Input: part model. Units: mm. Frame: model coordinates. Round coordinates to 2 decimals unless told otherwise and drop trailing zeros. Order: outer loops, then holes, each group sorted by start corner. A loop starts at its lowest first (then second) coordinate and runs counter-clockwise, first axis right, second up. Notation, with made-up numbers: (34, -29.75) -> (71, -29.75) arc R13 cw to (71, -11.75) -> close; hole circle Ø3 at (77.25, 69.25). An arc over 180 degrees is marked (long way). Use a Markdown table: item, result.
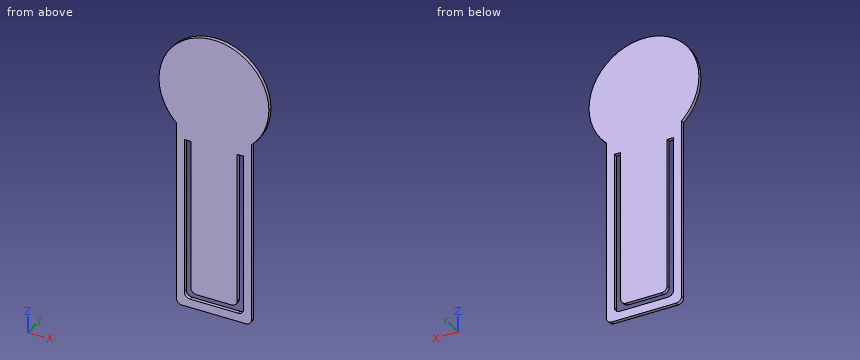
from build123d import *

# Parameters (mm, degrees)
F1_DEPTH = 1
F2_R     = 1.5
F3_R     = 1.5
F4_R     = 1.5
F5_R     = 1.5


with BuildPart() as f1:
    # F0 (on Front) → F1 (new body)
    with BuildSketch(Plane.XZ):
        with BuildLine():
            ThreePointArc((-12.582927, 26.823092), (-9.070294, 31.806561), (-7.831176, 37.776329))
            ThreePointArc((-7.831176, 37.776329), (-28.798743, 51.538165), (-33.082927, 26.826371))
            Line((-33.082927, 26.826371), (-12.582927, 26.826371))
            Line((-12.582927, 26.826371), (-12.582927, 26.823092))
        make_face()
        with BuildLine():
            Line((-12.582927, 26.826371), (-33.082927, 26.826371))
            ThreePointArc((-33.082927, 26.826371), (-22.833574, 22.776329), (-12.582927, 26.823092))
            Line((-12.582927, 26.823092), (-12.582927, 26.826371))
        make_face()
        with BuildLine():
            ThreePointArc((-12.582927, 26.823092), (-22.833574, 22.776329), (-33.082927, 26.826371))
            Line((-33.082927, 26.826371), (-33.082927, -23.173629))
            Line((-33.082927, -23.173629), (-12.582927, -23.173629))
            Line((-12.582927, -23.173629), (-12.582927, 26.823092))
        make_face()
        Polygon((-30.924927, -19.130884), (-30.924927, 22.876894), (-29.146819, 22.876894), (-29.146819, -19.130884), (-16.490985, -19.130884), (-16.490985, 23.022754), (-14.740985, 23.022754), (-14.740985, -19.130884), (-14.740985, -20.88121), (-16.490985, -20.88121), (-29.146819, -20.88121), (-30.924927, -20.88121), align=None, mode=Mode.SUBTRACT)
    extrude(amount=F1_DEPTH)

    # F2
    f2_edges = [f1.edges().sort_by_distance(p)[0] for p in [
        (-33.082927, -0.5, -23.173629),
        (-29.146819, -0.5, -19.130884),
    ]]
    fillet(f2_edges, radius=F2_R)

    # F3
    f3_edges = [f1.edges().sort_by_distance(p)[0] for p in [
        (-12.582927, -0.5, -23.173629),
        (-16.490985, -0.5, -19.130884),
    ]]
    fillet(f3_edges, radius=F3_R)

    # F4
    f4_edges = [f1.edges().sort_by_distance(p)[0] for p in [
        (-14.740985, -0.5, -20.88121),
    ]]
    fillet(f4_edges, radius=F4_R)

    # F5
    f5_edges = [f1.edges().sort_by_distance(p)[0] for p in [
        (-30.924927, -0.5, -20.88121),
    ]]
    fillet(f5_edges, radius=F5_R)


solid = f1.part
1) Cut plane B-B on y = -0.35. Return loops of the section in (x, z).
Results found:
| item | result |
|---|---|
| outline | (-33.08, -21.67) arc R1.5 ccw to (-31.58, -23.17) -> (-14.08, -23.17) arc R1.5 ccw to (-12.58, -21.67) -> (-12.58, 26.82) arc R15 ccw (long way) to (-33.08, 26.83) -> close; hole (-30.92, -19.38) arc R1.5 ccw to (-29.42, -20.88) -> (-16.24, -20.88) arc R1.5 ccw to (-14.74, -19.38) -> (-14.74, 23.02) -> (-16.49, 23.02) -> (-16.49, -17.63) arc R1.5 cw to (-17.99, -19.13) -> (-27.65, -19.13) arc R1.5 cw to (-29.15, -17.63) -> (-29.15, 22.88) -> (-30.92, 22.88) -> close |
2) Cut plane A-A on z = 6. Return loops of the section in (x, y).
Results found:
| item | result |
|---|---|
| outline | (-33.08, -1) -> (-30.92, -1) -> (-30.92, 0) -> (-33.08, 0) -> close; (-29.15, -1) -> (-16.49, -1) -> (-16.49, 0) -> (-29.15, 0) -> close; (-14.74, -1) -> (-12.58, -1) -> (-12.58, 0) -> (-14.74, 0) -> close |
3) Line query: L1, parallel to X at y = -0.15, z = 2; L2, parallel to Z at x = -21.5, y = -0.25; L3, parallel to Z at x = -26, y = -0.75. Output: solid intervals per line, ascending. Write a range as [from, to].
Results found:
| item | result |
|---|---|
| L1 | x = [-33.08, -30.92], [-29.15, -16.49], [-14.74, -12.58] |
| L2 | z = [-23.17, -20.88], [-19.13, 52.72] |
| L3 | z = [-23.17, -20.88], [-19.13, 52.44] |
4) Cut plane D-D on x = -36. Return loops of the section in (y, z).
Results found:
| item | result |
|---|---|
| outline | (-1, 30.59) -> (0, 30.59) -> (0, 44.96) -> (-1, 44.96) -> close |
5) Cut plane C-C on x = -15.5. Return loops of the section in (y, z), and give its area (3 significant figures).
Results found:
| item | result |
|---|---|
| outline | (-1, -23.17) -> (0, -23.17) -> (0, -20.69) -> (-1, -20.69) -> close; (-1, 23.02) -> (0, 23.02) -> (0, 50.86) -> (-1, 50.86) -> close |
| area | 30.3 mm² |
6) Pin query (flat end, axial travel): pin 1 Ø0.5 at (y, z) = (-0.5, 2.5) entering from -X. Return the tip coordinate at first contact, or that it passes through.
Results found:
| item | result |
|---|---|
| pin 1 | stops at x = -33.08 |
